Could you check a few things on this model? Use its own coordinates, in mm. Face numbers are marked on the shaded views. A direction names the side the tool comes from. Coordinates: 2 decimals unless noted, no trailing zeros. Write each loop counter-clockwise with the first axis right and the second up, starting at its lowest first coordinate (ties: lowest second). Pieces come first, ordered by that corner, then holes. Notation, with made-up numbers: M -6.5,-26 L 39.5,-26 A12 cw 39.5,-17 Z; hole C -10,-18 d11. An arc over 180 degrees is marked long. Write item = value, one per line.
```python
from build123d import *

# Parameters (mm, degrees)
SKETCH_1_W          = 17.8
SKETCH_1_H          = 42.8
EXTRUDE_1_DEPTH     = 5.5
SKETCH_2_R          = 6
EXTRUDE_2_DEPTH     = 12
EXTRUDE_START       = -12
SKETCH_3_R          = 6
EXTRUDE_3_DEPTH     = 12
SKETCH_4_R          = 3.60024343
CUT_EXTRUDE_1_DEPTH = 51
SKETCH_5_W          = 5.942865046
SKETCH_5_H          = 10.697157082
CUT_EXTRUDE_2_DEPTH = 18.8
SKETCH_6_R          = 2.15
CUT_EXTRUDE_3_DEPTH = 10
CUT_EXTRUDE_4_DEPTH = 3


with BuildPart() as part:
    # 草图1 → 凸台-拉伸1 (new body)
    with BuildSketch(Plane(origin=(0, 0, 0), x_dir=(1, 0, 0), z_dir=(0, 1, 0))):
        with Locations((8.9, -21.4)):
            Rectangle(SKETCH_1_W, SKETCH_1_H)
    extrude(amount=EXTRUDE_1_DEPTH)

    # 草图2 → 凸台-拉伸2 (add)
    with BuildSketch(Plane(origin=(0, 0, 0), x_dir=(-1, 0, 0), z_dir=(0, 0, -1))):
        with Locations((-17.8, 2.75)):
            Circle(SKETCH_2_R)
    extrude(amount=-EXTRUDE_2_DEPTH)

    # 草图3 → 凸台-拉伸3 (add)
    with BuildSketch(Plane.XY.offset(42.8).offset(EXTRUDE_START)):
        with Locations((17.8, 2.75)):
            Circle(SKETCH_3_R)
    extrude(amount=EXTRUDE_3_DEPTH)

    # 草图4 → 切除-拉伸1 (cut)
    with BuildSketch(Plane(origin=(0, 0, 0), x_dir=(-1, 0, 0), z_dir=(0, 0, -1))):
        with Locations((-17.8, 2.75)):
            Circle(SKETCH_4_R)
    extrude(amount=-CUT_EXTRUDE_1_DEPTH, mode=Mode.SUBTRACT)

    # 草图5 → 切除-拉伸2 (cut)
    with BuildSketch(Plane(origin=(0, 0, 30.8), x_dir=(-1, 0, 0), z_dir=(0, 0, -1))):
        with Locations((-14.980093676, 2.655560542)):
            Rectangle(SKETCH_5_W, SKETCH_5_H)
    extrude(amount=CUT_EXTRUDE_2_DEPTH, mode=Mode.SUBTRACT)

    # 草图6 → 切除-拉伸3 (cut)
    with BuildSketch(Plane(origin=(0, 5.5, 0), x_dir=(1, 0, 0), z_dir=(0, 1, 0))):
        with Locations(Location((5.420411498, -5.65, 0), (0, 0, 270))):
            Circle(SKETCH_6_R)
        with Locations(Location((5.420411498, -37.15, 0), (0, 0, 270))):
            Circle(SKETCH_6_R)
    extrude(amount=-CUT_EXTRUDE_3_DEPTH, mode=Mode.SUBTRACT)

    # 草图7 → 切除-拉伸4 (cut)
    with BuildSketch(Plane(origin=(0, 5.5, 0), x_dir=(1, 0, 0), z_dir=(0, 1, 0))):
        Polygon((2.920411498, -1.319872981), (7.920411498, -1.319872981), (10.420411498, -5.65), (7.920411498, -9.980127019), (2.920411498, -9.980127019), (0.420411498, -5.65), align=None)
        Polygon((0.420411498, -37.15), (2.920411498, -32.819872981), (7.920411498, -32.819872981), (10.420411498, -37.15), (7.920411498, -41.480127019), (2.920411498, -41.480127019), align=None)
    extrude(amount=-CUT_EXTRUDE_4_DEPTH, mode=Mode.SUBTRACT)


solid = part.part
```
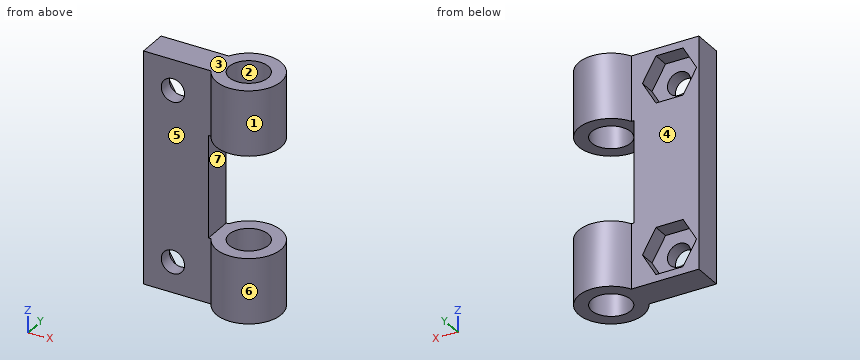
Item 1: For the marked faces 4, 5, 6 and 7, which set-ups out of +Z, -Z, +X, -X, +Y, -Y let a thin tool reach every point of the face, with its end or its side?
Numbers:
face_4 = +Z, -Z, -X, +Y
face_5 = +Z, -Z, -X, -Y
face_6 = +Z, -Z
face_7 = +X, +Y, -Y
Item 2: Imagine slicing it at C-C (z = 34). Write out the boundary of the cut face in (x, y).
Numbers:
outline = M 0,0 L 12.47,0 A6 ccw long 12.47,5.5 L 8.6,5.5 L 8.6,2.5 L 2.24,2.5 L 2.24,5.5 L 0,5.5 Z; hole C 17.8,2.75 d7.2
Item 3: If we mould it in two halves opening along X, with no side actions, what happens to the marked faces 1, 2 and 3? For each: pulls with the +X half, pulls with the -X half, needs draft (parallel to the pull), parting line crosses it, or undercut.
Numbers:
face_1 = parting line crosses it
face_2 = undercut
face_3 = needs draft
Item 4: Imagine slicing it at B-B (y = 1.5). Write out the boundary of the cut face in (x, z).
Numbers:
outline = M 0,0 L 14.42,0 L 14.42,12 L 12.01,12 L 12.01,30.8 L 14.42,30.8 L 14.42,42.8 L 0,42.8 Z; M 21.18,0 L 23.67,0 L 23.67,12 L 21.18,12 Z; M 21.18,30.8 L 23.67,30.8 L 23.67,42.8 L 21.18,42.8 Z; hole C 5.42,5.65 d4.3; hole C 5.42,37.15 d4.3
Item 5: I'm going to push flat-ended pins straight in: P1, Ø0.9, axis at x = 6.5, y = 4, coming from the -Z side; P2, Ø10, axis at x = 6, z = 19.5, coming from the -Y side; P3, Ø2.5, axis at x = 7, z = 37, coming from the +Y side; P4, Ø6, axis at x = 3.5, z = 20, coming from the +Y side. Where does each tip first touch, or does it pass through?
Numbers:
P1 = 0
P2 = 0
P3 = 2.5
P4 = 5.5
Item 6: Imagine slicing it at A-A (x = 17.8). Write out the boundary of the cut face in (y, z).
Numbers:
outline = M -3.25,0 L -0.85,0 L -0.85,12 L -3.25,12 Z; M -3.25,30.8 L -0.85,30.8 L -0.85,42.8 L -3.25,42.8 Z; M 6.35,0 L 8.75,0 L 8.75,12 L 6.35,12 Z; M 6.35,30.8 L 8.75,30.8 L 8.75,42.8 L 6.35,42.8 Z
Item 7: Imagine slicing it at D-D (y = -1.75). Write out the boundary of the cut face in (x, z).
Numbers:
outline = M 13.83,0 L 21.77,0 L 21.77,12 L 13.83,12 Z; M 13.83,30.8 L 21.77,30.8 L 21.77,42.8 L 13.83,42.8 Z
Item 8: If I drill on line 1 along Z through (x, y) = (4.75, 4.25); line 2 along Z through (x, y) = (6.25, 0.5); line 3 along Y through (x, z) = (17.75, 37.5), over which ranges is the centre line in solid material (lowest first)?
Numbers:
line_1 = 0 to 1.32, 9.98 to 32.82, 41.48 to 42.8
line_2 = 0 to 3.67, 7.63 to 35.17, 39.13 to 42.8
line_3 = -3.25 to -0.85, 6.35 to 8.75
